Could you check a few things on this model? Use its own coordinates, in mm. Face numbers are marked on the shaded views. Give positions to 0.01 mm unless a question says otherwise; leave off trailing zeros. Loops run counter-clockwise (first coordinate to the right, second up) from the corner with the lowest first, then second, coordinate; pieces in that order, holes last. Notation, with made-up numbers: (-9.5, -0.5) - (23.5, -0.5) arc R18 cw to (23.5, 10.5) - close; hole circle Ø7 at (-32, -16). An arc over 180 degrees is marked (long way). Write each question's results on one line, items separated by ' | '. Start each with the question number.
(1) Suppose I cut it at B-B (y = -6.5). Please give me the cut outline in (x, z).
(2) If we mould it in two halves opening along Y, with no side actions, what happens to the marked faces 1 and 2? For each: released by +Y, released by -Y, zero draft, split by the parting line, or undercut.
(3) For pin 1 (1.5 mm diameter, centred on y = 1.5, z = -142.5, fed in from -X); pin 2 (2.5 mm diameter, centred on x = 56.5, y = 1.5, fed in from -Z); pin 3 (3 mm diameter, centred on x = 51, y = -2.5, fed in from -Z); pin 4 (4 mm diameter, centred on x = 112, z = -43, fed in from -Y), each with a flat end and sliding along its axis, tell me the tip position at first contact or that it passes through.
(4) I need wall thicknesses on line 1 (X direction, y = -0.25, z = -133); line 2 (Y direction, x = 54.5, z = -74); line 3 (Z direction, x = 75, y = 2.75). Which ranges of each line are inside material? Lowest first, please.
(5) Suppose I cut it at D-D (z = -56). Please give me the cut outline in (x, y), and give its area (3 significant figures).
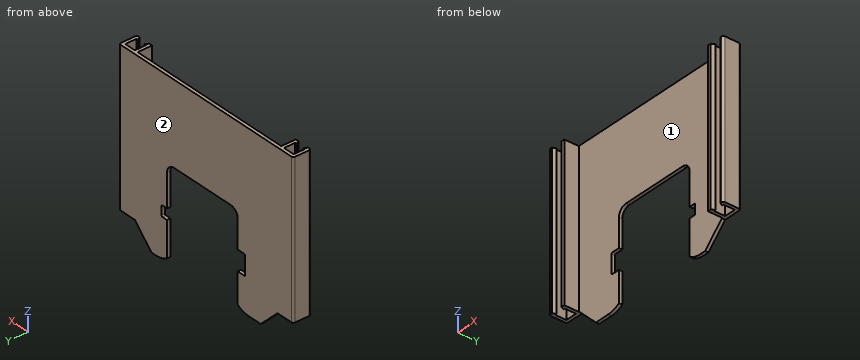
from build123d import *

# Parameters (mm, degrees)
SKETCH1_W           = 186.3
SKETCH1_H           = 72.76
BOSS_EXTRUDE1_DEPTH = 3
SKETCH3_W           = 59.3
SKETCH3_H           = 64
SKETCH3_W_2         = 51.35
BOSS_EXTRUDE3_DEPTH = 3
BOSS_EXTRUDE4_DEPTH = 3
CUT_EXTRUDE1_DEPTH  = 10
SKETCH9_W           = 3
SKETCH9_H           = 136.76
BOSS_EXTRUDE7_DEPTH = 13
FILLET1_R           = 7.5
BOSS_EXTRUDE8_DEPTH = 136.76
FILLET2_R           = 1.5


with BuildPart() as part:
    # Sketch1 → Boss-Extrude1 (new body)
    with BuildSketch(Plane(origin=(0, 0, 0), x_dir=(1, 0, 0), z_dir=(0, 1, 0))):
        with Locations((93.15, 36.38)):
            Rectangle(SKETCH1_W, SKETCH1_H)
    extrude(amount=BOSS_EXTRUDE1_DEPTH)

    # Sketch3 → Boss-Extrude3 (add)
    with BuildSketch(Plane(origin=(0, 3, 0), x_dir=(1, 0, 0), z_dir=(0, 1, 0))):
        with Locations((29.65, 104.76)):
            Rectangle(SKETCH3_W, SKETCH3_H)
        with Locations((160.625, 104.76)):
            Rectangle(SKETCH3_W_2, SKETCH3_H)
    extrude(amount=-BOSS_EXTRUDE3_DEPTH)

    # Sketch5 → Boss-Extrude4 (add)
    with BuildSketch(Plane(origin=(0, 3, 0), x_dir=(1, 0, 0), z_dir=(0, 1, 0))):
        with BuildLine():
            Line((169.56, 136.76), (151.56, 154.76))
            Line((151.56, 154.76), (146.56, 154.76))
            ThreePointArc((146.56, 154.76), (140.496954148, 153.865974954), (134.95, 151.26))
            Line((134.95, 151.26), (134.95, 136.76))
            Line((134.95, 136.76), (169.56, 136.76))
        make_face()
        with BuildLine():
            Line((59.3, 136.76), (16.69, 136.76))
            Line((16.69, 136.76), (34.69, 154.76))
            Line((34.69, 154.76), (47.69, 154.76))
            ThreePointArc((47.69, 154.76), (53.753045852, 153.865974954), (59.3, 151.26))
            Line((59.3, 151.26), (59.3, 136.76))
        make_face()
    extrude(amount=-BOSS_EXTRUDE4_DEPTH)

    # Sketch6 → Cut-Extrude1 (cut)
    with BuildSketch(Plane(origin=(0, 3, 0), x_dir=(1, 0, 0), z_dir=(0, 1, 0))):
        with BuildLine():
            Line((59.3, 123.76), (52.3, 123.76))
            ThreePointArc((52.3, 123.76), (51.592893219, 123.467106781), (51.3, 122.76))
            Line((51.3, 122.76), (51.3, 106.76))
            ThreePointArc((51.3, 106.76), (51.592893219, 106.052893219), (52.3, 105.76))
            Line((52.3, 105.76), (59.3, 105.76))
            Line((59.3, 105.76), (59.3, 123.76))
        make_face()
        with BuildLine():
            Line((139.95, 110.01), (134.95, 110.01))
            Line((134.95, 110.01), (134.95, 119.51))
            Line((134.95, 119.51), (139.95, 119.51))
            ThreePointArc((139.95, 119.51), (140.657106781, 119.217106781), (140.95, 118.51))
            Line((140.95, 118.51), (140.95, 111.01))
            ThreePointArc((140.95, 111.01), (140.657106781, 110.302893219), (139.95, 110.01))
        make_face()
    extrude(amount=-CUT_EXTRUDE1_DEPTH, mode=Mode.SUBTRACT)

    # Sketch9 → Boss-Extrude7 (add)
    with BuildSketch(Plane.XZ):
        with Locations((1.5, -68.38)):
            Rectangle(SKETCH9_W, SKETCH9_H)
        with Locations((184.8, -68.38)):
            Rectangle(SKETCH9_W, SKETCH9_H)
        with Locations((14.8, -68.38)):
            Rectangle(SKETCH9_W, SKETCH9_H)
        with Locations((171.5, -68.38)):
            Rectangle(SKETCH9_W, SKETCH9_H)
    extrude(amount=BOSS_EXTRUDE7_DEPTH)

    # Fillet1
    fillet1_edges = [part.edges().sort_by_distance(p)[0] for p in [
        (59.3, 1.5, -72.76),
        (134.95, 1.5, -72.76),
    ]]
    fillet(fillet1_edges, radius=FILLET1_R)

    # Sketch10 → Boss-Extrude8 (add)
    with BuildSketch(Plane(origin=(0, 0, -136.76), x_dir=(-1, 0, 0), z_dir=(0, 0, -1))):
        Polygon((-183.3, -13), (-181.8, -10), (-183.3, -10), align=None)
        Polygon((-174.5, -10), (-173, -10), (-173, -13), align=None)
        Polygon((-13.3, -10), (-13.3, -13), (-11.8, -10), align=None)
        Polygon((-4.5, -10), (-3, -10), (-3, -13), align=None)
    extrude(amount=-BOSS_EXTRUDE8_DEPTH)

    # Fillet2
    fillet2_edges = [part.edges().sort_by_distance(p)[0] for p in [
        (186.3, 3, -68.38),
        (0, -13, -68.38),
        (186.3, -13, -68.38),
        (0, 3, -68.38),
    ]]
    fillet(fillet2_edges, radius=FILLET2_R)


solid = part.part
Output values:
1) outline: (0, -136.76) - (3, -136.76) - (3, 0) - (0, 0) - close; (13.3, -136.76) - (16.3, -136.76) - (16.3, 0) - (13.3, 0) - close; (170, -136.76) - (173, -136.76) - (173, 0) - (170, 0) - close; (183.3, -136.76) - (186.3, -136.76) - (186.3, 0) - (183.3, 0) - close
2) face 1: released by -Y | face 2: released by +Y
3) pin 1: x = 21.68 | pin 2: z = -153.35 | pin 3: through | pin 4: y = 0
4) line 1: 0 to 3, 13.3 to 16.3, 170 to 173, 183.3 to 186.3 | line 2: 0 to 3 | line 3: -72.76 to 0
5) outline: (0, -11.5) arc R1.5 ccw to (1.5, -13) - (3, -13) - (4.5, -10) - (3, -10) - (3, 0) - (13.3, 0) - (13.3, -10) - (11.8, -10) - (13.3, -13) - (16.3, -13) - (16.3, 0) - (170, 0) - (170, -13) - (173, -13) - (174.5, -10) - (173, -10) - (173, 0) - (183.3, 0) - (183.3, -10) - (181.8, -10) - (183.3, -13) - (184.8, -13) arc R1.5 ccw to (186.3, -11.5) - (186.3, 1.5) arc R1.5 ccw to (184.8, 3) - (1.5, 3) arc R1.5 ccw to (0, 1.5) - close | area: 722 mm2
